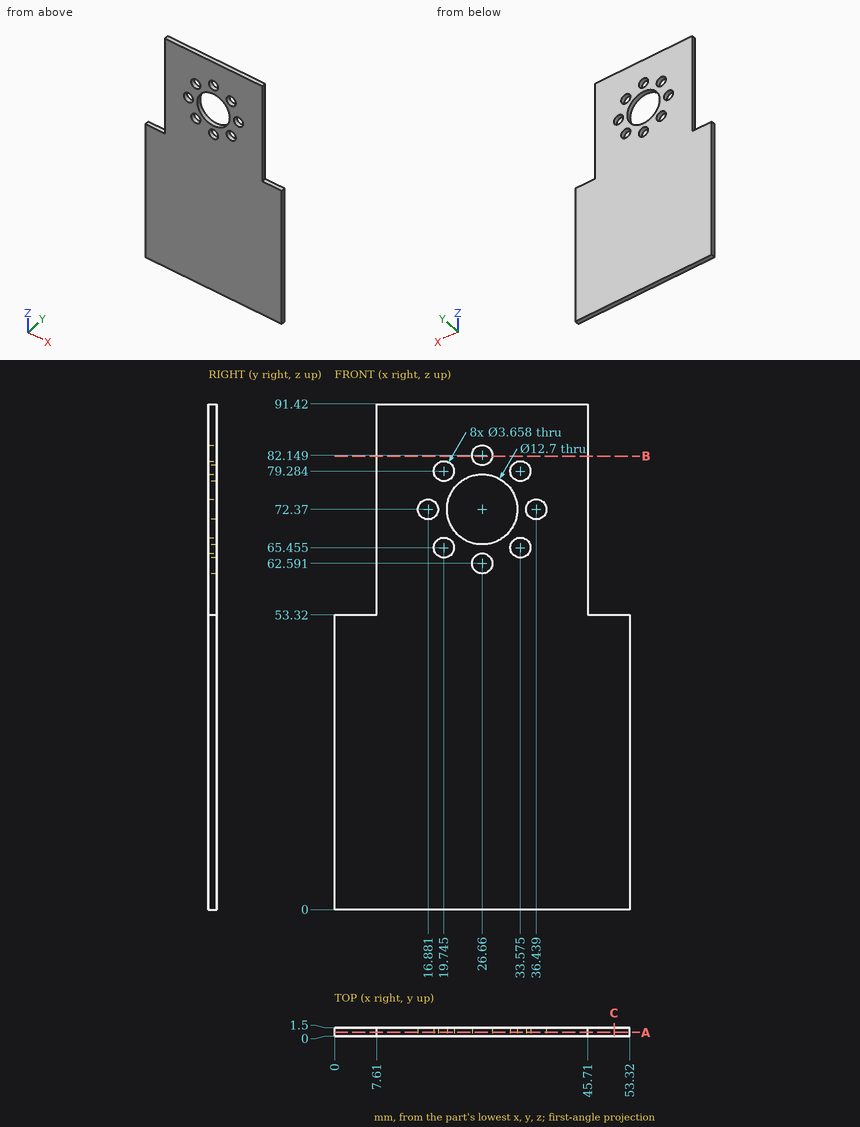
Can you work these out from the drawing? Everything is in mm from the part's minimum corner. Give positions to 0.01 mm unless a question says otherwise; leave off trailing zeros. Loops run counter-clockwise (first coordinate to the right, second up) from the corner with the lowest first, then second, coordinate; pieces in that order, holes last. Notation, with made-up numbers: (-22.75, -5.5) - (12.25, -5.5) arc R29 cw to (12.25, 18.5) - close; hole circle Ø6 at (42, 70.25). An arc over 180 degrees is marked (long way). Use one line per item in the form item = value.
1. I'm going to push flat-ended pins straight in: pin 1 Ø3 at (x, z) = (33.57, 79.28) entering from +Y; pin 2 Ø0.8 at (x, y) = (2.5, 0.5) entering from +Z. Where does each tip first touch, or does it pass through?
Response values:
pin_1 = through
pin_2 = 53.32
2. I want a section at A-A (y = 0.65). Give the number of separate pieces and of enclosed holes in the cut face, and give its area (3 significant figures).
Response values:
separate_pieces = 1
enclosed_holes = 9
area = 4,080 mm²
3. I want a section at B-B (z = 82). Please give me the cut outline in (x, y).
Response values:
outline = (7.61, 0) - (24.84, 0) - (24.84, 1.5) - (7.61, 1.5) - close; (28.48, 0) - (45.71, 0) - (45.71, 1.5) - (28.48, 1.5) - close
4. I need wall thicknesses on probe 1 along X at (y, z) = (0.4, 79); probe 2 along Z at (x, y) = (32.5, 0.15) (1 decimal); probe 3 along Z at (x, y) = (25, 1.4) (1 decimal). Which ranges of each line are inside material? Lowest first, please.
Response values:
probe_1 = 7.61 to 17.94, 21.55 to 31.77, 35.38 to 45.71
probe_2 = 0 to 64, 66.9 to 69.9, 74.9 to 77.8, 80.8 to 91.4
probe_3 = 0 to 61.8, 63.4 to 66.2, 78.5 to 81.4, 82.9 to 91.4
5. I want a section at C-C (x = 50.5). Please give me the cut outline in (y, z).
Response values:
outline = (0, 0) - (1.5, 0) - (1.5, 53.32) - (0, 53.32) - close
